from build123d import *

# Parameters (mm, degrees)
SKETCH1_R           = 3
BOSS_EXTRUDE1_DEPTH = 3.1
SKETCH2_R           = 2.5
CUT_EXTRUDE1_DEPTH  = 4.1
SKETCH3_W           = 37.5
SKETCH3_H           = 3.1
CUT_EXTRUDE2_DEPTH  = 4.1
SKETCH7_R           = 3.25
CUT_EXTRUDE5_DEPTH  = 4.1


with BuildPart() as part:
    # Sketch1 → Boss-Extrude1 (new body)
    with BuildSketch(Plane.XY):
        with BuildLine():
            Line((0, -47.625), (251.196924141, -47.625))
            Line((251.196924141, -47.625), (251.196924141, 47.609956917))
            Line((251.196924141, 47.609956917), (1.196924141, 47.609956917))
            ThreePointArc((1.196924141, 47.609956917), (-47.621239081, 0.598509335), (0, -47.625))
        make_face()
        with Locations((0, -41.275)):
            Circle(SKETCH1_R, mode=Mode.SUBTRACT)
        with Locations((-41.275, 0)):
            Circle(SKETCH1_R, mode=Mode.SUBTRACT)
        with Locations((0, 41.275)):
            Circle(SKETCH1_R, mode=Mode.SUBTRACT)
        with Locations((41.275, 0)):
            Circle(SKETCH1_R, mode=Mode.SUBTRACT)
    extrude(amount=BOSS_EXTRUDE1_DEPTH)

    # Sketch2 → Cut-Extrude1 (cut, through all)
    with BuildSketch(Plane.XY.offset(3.1)):
        with Locations((-19.445436483, 7.071067812)):
            Circle(SKETCH2_R)
        with Locations((-7.071067812, 19.445436483)):
            Circle(SKETCH2_R)
        with Locations((40.658639918, -28.284271247)):
            Circle(SKETCH2_R)
        with Locations((28.284271247, -40.658639918)):
            Circle(SKETCH2_R)
        Polygon((21.213203436, -42.072853481), (42.072853481, -21.213203436), (0, 20.859650045), (-20.859650045, 0), align=None)
    extrude(amount=-CUT_EXTRUDE1_DEPTH, mode=Mode.SUBTRACT)

    # Sketch3 → Cut-Extrude2 (cut, through all)
    with BuildSketch(Plane.XY.offset(3.1)):
        with Locations((232.446924141, -46.075)):
            Rectangle(SKETCH3_W, SKETCH3_H)
    cut_extrude2 = extrude(amount=-CUT_EXTRUDE2_DEPTH, mode=Mode.SUBTRACT)

    # Mirror1: Cut-Extrude2 across plane
    add(cut_extrude2.mirror(Plane.ZX), mode=Mode.SUBTRACT)

    # Sketch7 → Cut-Extrude5 (cut, through all)
    with BuildSketch(Plane.XY.offset(3.1)):
        with Locations((226.196924141, -30.525)):
            Circle(SKETCH7_R)
        with Locations((226.196924141, -7.525)):
            Circle(SKETCH7_R)
        with Locations((226.196924141, 7.525)):
            Circle(SKETCH7_R)
        with Locations((226.196924141, 30.525)):
            Circle(SKETCH7_R)
        with Locations((201.196924141, -30.525)):
            Circle(SKETCH7_R)
        with Locations((201.196924141, -7.525)):
            Circle(SKETCH7_R)
        with Locations((201.196924141, 7.525)):
            Circle(SKETCH7_R)
        with Locations((201.196924141, 30.525)):
            Circle(SKETCH7_R)
    extrude(amount=-CUT_EXTRUDE5_DEPTH, mode=Mode.SUBTRACT)


solid = part.part
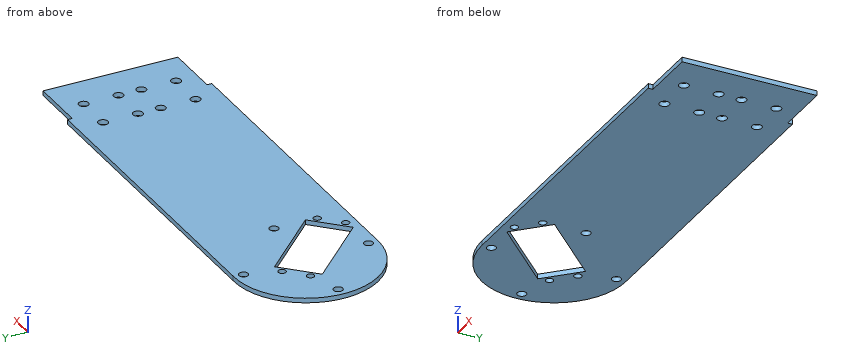
Verification items for the finished model (mm, model axes). Coordinates: 2 decimals unless noted, no trailing zeros. Order: outer loops, then holes, each group sorted by start corner. A loop starts at its lowest first (then second) coordinate and runs counter-clockwise, first axis right, second up.
1. Sectioned sample at A-A, the plane y = 14. Record the cut outline in (x, z).
Results found:
outline: (-45.52, 0) - (-6.86, 0) - (-6.86, 3.1) - (-45.52, 3.1) - close; (6.86, 0) - (251.2, 0) - (251.2, 3.1) - (6.86, 3.1) - close
2. Scan lines: line 1 (Y direction, x = 0, z = 1.7) (3 decimals); line 2 (X direction, y = -5, z = 2.55); line 3 (X direction, y = 10, z = 1.15). Record each from-to range of solid material in increasing order.
Results found:
line 1: y = -47.625 to -44.275, -38.275 to -20.86, 20.86 to 38.275, 44.275 to 47.625
line 2: x = -47.36 to -15.86, 25.86 to 199.15, 203.24 to 224.15, 228.24 to 251.2
line 3: x = -46.56 to -10.86, 10.86 to 199.09, 203.3 to 224.09, 228.3 to 251.2
3. Go/stop test with flat-tipped pins: pin 1 Ø1 at (y, z) = (-20, 1.5) entering from -X; pin 2 Ø1.5 at (x, z) = (-14.5, 1.5) entering from +Y; pin 3 Ø0.9 at (y, z) = (45.5, 2) entering from +X. Record where each tip stops, or that it passes through.
Results found:
pin 1: stops at x = -43.45
pin 2: stops at y = 45.6
pin 3: stops at x = 213.7
4. Sectioned sample at B-B, the plane z = 1. Give the number of separate pieces and of enclosed holes in the cut face, and give its area (3 significant figures).
Results found:
separate pieces: 1
enclosed holes: 17
area: 25,000 mm2
